```python
from build123d import *

# Parameters (mm, degrees)
F0_R          = 8
F1_DEPTH      = 10
F2_R          = 6
F3_DEPTH      = 13
F3_DEPTH_BACK = 3
F5_DEPTH      = 10
F13_R         = 1.5
F16_DEPTH     = 3
F14_R         = 1.5
F17_DEPTH     = 3
F15_R         = 1.5
F18_DEPTH     = 3
F6_R          = 1.5
F19_DEPTH     = 3
F7_R          = 1.5
F20_DEPTH     = 3
F8_R          = 1.5
F21_DEPTH     = 3
F9_R          = 1.5
F22_DEPTH     = 3
F10_R         = 1.5
F23_DEPTH     = 3
F11_R         = 1.5
F24_DEPTH     = 3
F12_R         = 1.5
F25_DEPTH     = 3
F26_R         = 3
F27_DEPTH     = 16
F28_R         = 9.2657382737
F28_R_2       = 8
F29_DEPTH     = 10
F30_R         = 1


with BuildPart() as f1:
    # F0 (on Front) → F1 (new body)
    with BuildSketch(Plane.XZ):
        Circle(F0_R)
    extrude(amount=F1_DEPTH)

    # F2 (on face) → F3 (join, two sides)
    with BuildSketch(Plane(origin=(0, 0, 0), x_dir=(-1, 0, 0), z_dir=(0, 1, 0))) as f3_sk:
        Circle(F2_R)
    extrude(amount=-F3_DEPTH)
    extrude(f3_sk.sketch, amount=F3_DEPTH_BACK)

    # F4 (on Front) → F5 (join)
    with BuildSketch(Plane.XZ):
        Polygon((-8.2126331182, -1.8191528364), (-5.5748885523, -6.2989901894), (-0.8077260429, -8.3728273848), (4.2679603613, -7.2485291012), (7.7134309701, -3.3555390694), (8.2126331182, 1.8191528364), (5.5748885523, 6.2989901894), (0.8077260429, 8.3728273848), (-4.2679603613, 7.2485291012), (-7.7134309701, 3.3555390694), align=None)
    extrude(amount=F5_DEPTH)

    # F13 (on face) → F16 (cut)
    with BuildSketch(Plane(origin=(7.9630320441, 0, -0.7681931165), x_dir=(0, 1, 0), z_dir=(0.9953790055, 0, -0.0960241396))):
        with Locations((-5, 0)):
            Circle(F13_R)
    extrude(amount=-F16_DEPTH, mode=Mode.SUBTRACT)

    # F14 (on face) → F17 (cut)
    with BuildSketch(Plane(origin=(6.8937608352, 0, 4.0590715129), x_dir=(0, 1, 0), z_dir=(0.8617201044, 0, 0.5073839391))):
        with Locations((-5, 0)):
            Circle(F14_R)
    extrude(amount=-F17_DEPTH, mode=Mode.SUBTRACT)

    # F15 (on face) → F18 (cut)
    with BuildSketch(Plane(origin=(3.1913072976, 0, 7.3359087871), x_dir=(0.9169885984, 0, -0.3989134122), z_dir=(0.3989134122, 0, 0.9169885984))):
        with Locations((0, -5)):
            Circle(F15_R)
    extrude(amount=-F18_DEPTH, mode=Mode.SUBTRACT)

    # F6 (on face) → F19 (cut)
    with BuildSketch(Plane(origin=(-1.7301171592, 0, 7.810678243), x_dir=(0.9763347804, 0, 0.2162646449), z_dir=(-0.2162646449, 0, 0.9763347804))):
        with Locations((0, -5)):
            Circle(F6_R)
    extrude(amount=-F19_DEPTH, mode=Mode.SUBTRACT)

    # F7 (on face) → F20 (cut)
    with BuildSketch(Plane(origin=(-5.9906956657, 0, 5.3020340853), x_dir=(0, -1, 0), z_dir=(-0.7488369582, 0, 0.6627542607))):
        with Locations((5, 0)):
            Circle(F7_R)
    extrude(amount=-F20_DEPTH, mode=Mode.SUBTRACT)

    # F8 (on face) → F21 (cut)
    with BuildSketch(Plane(origin=(-7.9630320441, 0, 0.7681931165), x_dir=(0, -1, 0), z_dir=(-0.9953790055, 0, 0.0960241396))):
        with Locations((5, 0)):
            Circle(F8_R)
    extrude(amount=-F21_DEPTH, mode=Mode.SUBTRACT)

    # F9 (on face) → F22 (cut)
    with BuildSketch(Plane(origin=(-6.8937608352, 0, -4.0590715129), x_dir=(0, -1, 0), z_dir=(-0.8617201044, 0, -0.5073839391))):
        with Locations((5, 0)):
            Circle(F9_R)
    extrude(amount=-F22_DEPTH, mode=Mode.SUBTRACT)

    # F10 (on face) → F23 (cut)
    with BuildSketch(Plane(origin=(-3.1913072976, 0, -7.3359087871), x_dir=(0.9169885984, 0, -0.3989134122), z_dir=(-0.3989134122, 0, -0.9169885984))):
        with Locations((0, 5)):
            Circle(F10_R)
    extrude(amount=-F23_DEPTH, mode=Mode.SUBTRACT)

    # F11 (on face) → F24 (cut)
    with BuildSketch(Plane(origin=(1.7301171592, 0, -7.810678243), x_dir=(0.9763347804, 0, 0.2162646449), z_dir=(0.2162646449, 0, -0.9763347804))):
        with Locations((0, 5)):
            Circle(F11_R)
    extrude(amount=-F24_DEPTH, mode=Mode.SUBTRACT)

    # F12 (on face) → F25 (cut)
    with BuildSketch(Plane(origin=(5.9906956657, 0, -5.3020340853), x_dir=(0, 1, 0), z_dir=(0.7488369582, 0, -0.6627542607))):
        with Locations((-5, 0)):
            Circle(F12_R)
    extrude(amount=-F25_DEPTH, mode=Mode.SUBTRACT)

    # F26 (on face) → F27 (cut)
    with BuildSketch(Plane(origin=(0, 3, 0), x_dir=(-1, 0, 0), z_dir=(0, 1, 0))):
        Circle(F26_R)
    extrude(amount=-F27_DEPTH, mode=Mode.SUBTRACT)

    # F28 (on Front) → F29 (cut)
    with BuildSketch(Plane.XZ):
        Circle(F28_R)
        Circle(F28_R_2, mode=Mode.SUBTRACT)
    extrude(amount=F29_DEPTH, mode=Mode.SUBTRACT)

    # F30
    f30_edges = [f1.edges().sort_by_distance(p)[0] for p in [
        (-8, -10, 0),
        (6, -13, 0),
        (-8, 0, 0),
        (6, 3, 0),
    ]]
    fillet(f30_edges, radius=F30_R)


solid = f1.part
```
Build history of the part. All positions in model axes, mm. A direction names the side the tool comes from. Round coordinates to 2 decimals unless told otherwise and drop trailing zeros. Use a Markdown table: item, result.
1) Pull direction Z, two halves, no side cores. Call faces 1 (the face through (0.1, 3, -3.3)), 2 (the face through (6, -11, 0)), 3 (the face through (3.913, -4.549, 5.409)): pulls with the +Z half, pulls with the -Z half, needs draft (parallel to the pull), parting line crosses it, or undercut.
Recorded:
| item | result |
|---|---|
| face 1 | needs draft |
| face 2 | parting line crosses it |
| face 3 | undercut |
2) Flat gauge pins, fed straight in: pin 1 Ø3 at (y, z) = (-3, -5) entering from -X; pin 2 Ø3 at (x, y) = (3, -0.5) entering from -Z; pin 3 Ø2 at (y, z) = (-9.5, -3.5) entering from -X. Where does each tip first touch, or does it go through?
Recorded:
| item | result |
|---|---|
| pin 1 | stops at x = -7.19 |
| pin 2 | stops at z = -7.84 |
| pin 3 | stops at x = -7.57 |
3) Wall check: L1, parallel to Z at x = 0, y = -8.5; L2, parallel to Y at x = -2.5, z = -5.75; L3, parallel to Y at x = 1.25, z = -5.25. Give the ranges that are in metal, low to high.
Recorded:
| item | result |
|---|---|
| L1 | z = -8 to -3, 3 to 8 |
| L2 | y = -10 to -6.5, -3.5 to 0 |
| L3 | y = -12.92 to -6.5, -3.5 to 2.92 |
4) Tool access for faces 4 (the face through (6, 0, 2)), 5 (the face through (4.298, -5.021, 2.555)), 6 (the face through (7.39, -4.94, -3.06)): list every direction of +Z, -Z, +X, -X, +Y, -Y with a clear straight run to the whole face (end or side of a thin tool).
Recorded:
| item | result |
|---|---|
| face 4 | +Y |
| face 5 | none |
| face 6 | +Y, -Y |
5) Saw through at A-A on x = 0. Give the number of separate pieces and of enclosed holes in the cut face, and give its area (3 significant figures).
Recorded:
| item | result |
|---|---|
| separate pieces | 2 |
| enclosed holes | 2 |
| area | 129 mm² |
